Geometry check sheet. Reference: the model listing, model coordinates, mm. A direction names the side the tool comes from. Give positions to 0.01 mm unless a question says otherwise; leave off trailing zeros. Write each loop counter-clockwise with the first axis right and the second up, starting at its lowest first coordinate (ties: lowest second). Pieces come first, ordered by that corner, then holes.
(1) Thickness scan on line 1 along Z through (x, y) = (-17, -9.5); line 2 along Z through (x, y) = (-2.5, -1); line 3 along Y through (x, z) = (-0.5, 21). Record the ranges inside material, lowest first.
(2) Mould release check, pull along Y, two halves, no side actions. Record for faces 4 (the flat face through (4.294, -14.794, 18.741)), 5 (the flat face through (-12.22, -20.82, 32.96)), 6 (the flat face through (0, 0, 48)), 7 (the flat face through (12.22, 20.82, 32.96)): +Y half, -Y half, draft (parallel to the pull), parting line (faces both ways), or undercut.
(3) Depth check by flat-ended pin: P1, Ø6, axis at y = 17.5, z = 34.5, coming from the +X side; P2, Ø4, axis at x = 1.5, y = 18.5, coming from the -Z side; P3, Ø6, axis at x = -8, y = -9.5, coming from the -Z side. Enter the tip coordinate at first touch or a pass-through.
(4) Cross-section at C-C (x = -21.5). Record the boundary of the cut face in (y, z).
(5) Cross-section at A-A (z = 44). Record the boundary of the cut face in (x, y), and give its area (3 significant figures).
(6) Tool access check on faces 1 (the flat face through (0, 0, 24.142)), 2 (the flat face through (-3.7, 15.2, 18.5)), 3 (the flat face through (-20.82, 12.22, 32.96)). Record the directions out of +Z, -Z, +X, -X, +Y, -Y that give a thin tool (end or side, any length) a straight path to the whole face; none if there is none.
(7) Cross-section at D-D (x = 23). Record the boundary of the cut face in (y, z).
(8) Cross-section at B-B (z = 39). Record the boundary of the cut face in (x, y).
```python
from build123d import *

# Parameters (mm, degrees)
F1_DEPTH = 48
F2_W     = 20
F2_H     = 24.1421356237
F3_DEPTH = 55.8448557599
F4_R     = 7.4299584593
F5_DEPTH = 55.8448557599


with BuildPart() as f1:
    # F0 (on Top) → F1 (new body)
    with BuildSketch(Plane.XY):
        Polygon((-15.8813725217, 20.7514992061), (-25.9033520131, 3.4436996038), (-20.7514992061, -15.8813725217), (-3.4436996038, -25.9033520131), (15.8813725217, -20.7514992061), (25.9033520131, -3.4436996038), (20.7514992061, 15.8813725217), (3.4436996038, 25.9033520131), align=None)
    extrude(amount=F1_DEPTH)

    # F2 (on face) → F3 (cut, through all)
    with BuildSketch(Plane(origin=(23.3274256096, 6.218836459, 0), x_dir=(-0.2575926403, 0.9662536063, 0), z_dir=(0.9662536063, 0.2575926403, 0))):
        Polygon((-10, 24.1421356237), (-24.1421356237, 10), (-24.1421356237, -10), (-10, -24.1421356237), (10, -24.1421356237), (24.1421356237, -10), (24.1421356237, 10), (10, 24.1421356237), (10, 0), (-10, 0), align=None)
        with Locations((0, 12.0710678119)):
            Rectangle(F2_W, F2_H)
    extrude(amount=-F3_DEPTH, mode=Mode.SUBTRACT)

    # F4 (on face) → F5 (cut, through all)
    with BuildSketch(Plane(origin=(6.218836459, -23.3274256096, 0), x_dir=(0.9662536063, 0.2575926403, 0), z_dir=(0.2575926403, -0.9662536063, 0))):
        with Locations((1.4277122682, 35.5290137231)):
            Circle(F4_R)
    extrude(amount=-F5_DEPTH, mode=Mode.SUBTRACT)


solid = f1.part
```
Reply:
1. line 1: z = 24.14 to 48
1. line 2: z = 24.14 to 29.33, 41.72 to 48
1. line 3: y = -25.12 to -13.73, 13.47 to 24.85
2. face 4: undercut
2. face 5: -Y half
2. face 6: draft
2. face 7: +Y half
3. P1: stops at x = 21.12
3. P2: stops at z = 14.65
3. P3: stops at z = 24.02
4. outline: (-13.07, 24.14) - (4.62, 24.14) - (11.05, 17.93) - (11.05, 48) - (-13.07, 48) - close
5. outline: (-25.9, 3.44) - (-20.75, -15.88) - (-3.44, -25.9) - (15.88, -20.75) - (25.9, -3.44) - (20.75, 15.88) - (3.44, 25.9) - (-15.88, 20.75) - close
5. area: 1,930 mm2
6. face 1: -Z
6. face 2: -Z, +X
6. face 3: +Z, -Z, -X, +Y
7. outline: (-8.46, 20.05) - (-4.22, 24.14) - (7.45, 24.14) - (7.45, 48) - (-8.46, 48) - close
8. outline: (-25.9, 3.44) - (-20.75, -15.88) - (-3.44, -25.9) - (1.25, -24.65) - (-11.19, 22) - (-15.88, 20.75) - close; (1.51, 25.39) - (13.95, -21.27) - (15.88, -20.75) - (25.9, -3.44) - (20.75, 15.88) - (3.44, 25.9) - close
